Check sheet for the modelled part. Datum: model origin and axes. Units: mm. A direction names the side the tool comes from. Round coordinates to 2 decimals unless told otherwise and drop trailing zeros. Write each loop counter-clockwise with the first axis right and the second up, starting at its lowest first coordinate (ties: lowest second). Pieces come first, ordered by that corner, then holes.
Item 1: Cross-section at D-D on x = -7.5. Enter the section's corners in (y, z), plus the area to 3 significant figures.
Item 2: Tool access check on faces 1 (the flat face through (15.393, -6.418, 42.675)), 2 (the flat face through (-12.528, -13, 27)), 3 (the flat face through (15.025, 6.218, 42.675)), 4 (the flat face through (15.53, -4.61, 39.86)). Record the directions out of +Z, -Z, +X, -X, +Y, -Y that give a thin tool (end or side, any length) a straight path to the whole face; none if there is none.
Item 3: Release check for a two-part mould opening along Y. For faces 5 (the flat face through (12.472, -13, 27)), 6 (the flat face through (0, -25, 27)), 7 (the cylindrical face through (6, 0, 53)) record: +Y half, -Y half, draft (parallel to the pull), parting line (faces both ways), or undercut.
Item 4: Material ranges on line 1 (X direction, y = 2, z = 40.5); line 2 (Y direction, x = 0, z = 51.9); line 3 (X direction, y = 1, z = 3), recorded low to high.
Item 5: Cross-section at B-B on x = 0. Enter the section's corners in (y, z), plus the area to 4 significant figures.
Item 6: Cross-section at A-A on z = 43. Count the separate pieces of the cut face and the enclosed holes in it, plus the area to 3 significant figures.
Item 7: Go/stop test with flat-tipped pins: pin 1 Ø17 at (x, y) = (-1, -2) entering from -Z; pin 2 Ø3 at (y, z) = (1, 38.5) entering from +X; pin 3 Ø9.5 at (x, y) = (0, 0) entering from -Z; pin 4 Ø10 at (x, z) = (19.5, 36.5) entering from -Y. Record where each tip stops, or that it passes through.
from build123d import *

# Parameters (mm, degrees)
F7_R     = 12.5
F0_DEPTH = 55
F1_W     = 25
F1_H     = 25
F8_DEPTH = 55
F2_D     = 12
F10_R    = 10.5
F3_DEPTH = 50
F5_DEPTH = 25
F6_DEPTH = 20


with BuildPart() as f0:
    # F7 (on Top) → F0 (new body)
    with BuildSketch(Plane.XY):
        Circle(F7_R)
    extrude(amount=F0_DEPTH)

    # F1 (on Top) → F8 (join)
    with BuildSketch(Plane.XY):
        with Locations((-0.0282753837, -12.5)):
            Rectangle(F1_W, F1_H)
    extrude(amount=F8_DEPTH)

    # F2 (through all)
    with Locations(Plane(origin=(0, 0, 0), x_dir=(1, 0, 0), z_dir=(0, 0, -1))):
        with Locations((0, 0)):
            Hole(F2_D / 2)

    # F10 (on Top) → F3 (cut)
    with BuildSketch(Plane.XY):
        Circle(F10_R)
    extrude(amount=F3_DEPTH, mode=Mode.SUBTRACT)

    # F11 (on face) → F5 (join)
    with BuildSketch(Plane.XY.offset(55)):
        with BuildLine():
            Line((12.4717246163, -4.7753756192), (18.3970628421, -8.107226411))
            Line((18.3970628421, -8.107226411), (25.3720879555, -3.9738714695))
            Line((25.3720879555, -3.9738714695), (25.28001013, 4.1333549415))
            Line((25.28001013, 4.1333549415), (18.2129071911, 8.107226411))
            Line((18.2129071911, 8.107226411), (11.7462114787, 4.2751041973))
            ThreePointArc((11.7462114787, 4.2751041973), (12.3761431106, 1.7553010303), (12.4717246163, -0.8402886979))
            Line((12.4717246163, -0.8402886979), (12.4717246163, -4.7753756192))
        make_face()
    extrude(amount=-F5_DEPTH)

    # F12 (on face) → F6 (cut)
    with BuildSketch(Plane(origin=(0, 0, 30), x_dir=(1, 0, 0), z_dir=(0, 0, -1))):
        Polygon((12.8416223451, -3.0601453381), (18.1419495493, -6.1202906762), (23.4422767535, -3.0601453381), (23.4422767535, 3.0601453381), (18.1419495493, 6.1202906762), (12.8416223451, 3.0601453381), align=None)
    extrude(amount=-F6_DEPTH, mode=Mode.SUBTRACT)


solid = f0.part
Response values:
1. outline: (-25, 0) - (-7.35, 0) - (-7.35, 50) - (7.35, 50) - (7.35, 0) - (10, 0) - (10, 55) - (-25, 55) - close
1. area: 1,190 mm2
2. face 1: +Z, -Z, -Y
2. face 2: +Z, -Z, -X, +Y, -Y
2. face 3: +Z, -Z, +Y
2. face 4: -Z
3. face 5: draft
3. face 6: -Y half
3. face 7: undercut
4. line 1: x = -12.34 to -10.31, 10.31 to 12.84, 23.44 to 25.3
4. line 2: y = -25 to -6, 6 to 12.5
4. line 3: x = -12.46 to -10.45, 10.45 to 12.46
5. outline: (-25, 0) - (-10.5, 0) - (-10.5, 50) - (-6, 50) - (-6, 55) - (-25, 55) - close; (6, 50) - (10.5, 50) - (10.5, 0) - (12.5, 0) - (12.5, 55) - (6, 55) - close
5. area: 952.5 mm2
6. separate pieces: 1
6. enclosed holes: 2
6. area: 588 mm2
7. pin 1: stops at z = 0
7. pin 2: stops at x = 25.33
7. pin 3: passes through
7. pin 4: stops at y = -8.11
